Model file for the job. Use its own axes, mm. A direction names the side the tool comes from. Give positions to 0.01 mm unless a question says otherwise; leave off trailing zeros. Write each loop counter-clockwise with the first axis right and the second up, starting at its lowest first coordinate (ties: lowest second). Pieces come first, ordered by that corner, then holes.
```python
from build123d import *

# Parameters (mm, degrees)
BOSS_EXTRUDE1_DEPTH = 6.35
CUT_EXTRUDE1_DEPTH  = 64.001230115
FILLET2_R           = 3.81


with BuildPart() as part:
    # Sketch1 → Boss-Extrude1 (new body)
    with BuildSketch(Plane.XY):
        with BuildLine():
            Line((0, 47.625), (0, 36.83))
            ThreePointArc((0, 36.83), (36.83, 0), (0, -36.83))
            add(Edge.make_bspline(
                [(0, 47.625), (-26.600153249, 47.625), (-56.149642057, -0.404637175), (-24.15519568, -36.984078787), (0, -36.83)],
                knots=[0, 0, 0, 0, 0.529165327, 1, 1, 1, 1], degree=3))
        make_face()
        with BuildLine():
            Line((1.1176, -8.255), (8.255, -8.255))
            Line((8.255, -8.255), (8.255, -1.1176))
            Line((8.255, -1.1176), (9.657085657, -1.1176))
            ThreePointArc((9.657085657, -1.1176), (14.478, 0), (9.657085657, 1.1176))
            Line((9.657085657, 1.1176), (8.255, 1.1176))
            Line((8.255, 1.1176), (8.255, 8.255))
            Line((8.255, 8.255), (1.1176, 8.255))
            Line((1.1176, 8.255), (1.1176, 9.657085657))
            ThreePointArc((1.1176, 9.657085657), (0, 14.478), (-1.1176, 9.657085657))
            Line((-1.1176, 9.657085657), (-1.1176, 8.255))
            Line((-1.1176, 8.255), (-8.255, 8.255))
            Line((-8.255, 8.255), (-8.255, 1.1176))
            Line((-8.255, 1.1176), (-9.657085657, 1.1176))
            ThreePointArc((-9.657085657, 1.1176), (-14.478, 0), (-9.657085657, -1.1176))
            Line((-9.657085657, -1.1176), (-8.255, -1.1176))
            Line((-8.255, -1.1176), (-8.255, -8.255))
            Line((-8.255, -8.255), (-1.1176, -8.255))
            Line((-1.1176, -8.255), (-1.1176, -9.657085657))
            ThreePointArc((-1.1176, -9.657085657), (0, -14.478), (1.1176, -9.657085657))
            Line((1.1176, -9.657085657), (1.1176, -8.255))
        make_face(mode=Mode.SUBTRACT)
    extrude(amount=BOSS_EXTRUDE1_DEPTH)

    # Sketch5 → Cut-Extrude1 (cut, through all)
    with BuildSketch(Plane.XY.offset(6.35)):
        with BuildLine():
            ThreePointArc((-12.136378722, 32.883902073), (-23.899090909, 25.641297895), (-31.950108913, 14.416422734))
            ThreePointArc((-31.950108913, 14.416422734), (-28.392549398, 5.00872066), (-18.984847325, 8.566280175))
            ThreePointArc((-18.984847325, 8.566280175), (-14.200909091, 15.236133532), (-7.211471414, 19.539709927))
            ThreePointArc((-7.211471414, 19.539709927), (-3.001828995, 28.674259654), (-12.136378722, 32.883902073))
        make_face()
    extrude(amount=-CUT_EXTRUDE1_DEPTH, mode=Mode.SUBTRACT)

    # Fillet2
    fillet2_edges = [part.edges().sort_by_distance(p)[0] for p in [
        (0, 36.83, 3.175),
    ]]
    fillet(fillet2_edges, radius=FILLET2_R)


solid = part.part
```
1. Slice it at B-B, the plane z = 4.75. State how many separate pieces and enclosed holes the cut face has, and give its area (3 significant figures).
Calculated:
separate pieces: 1
enclosed holes: 2
area: 4,020 mm2
2. Pin check, flat tips, straight feed: P1, Ø2, axis at y = 10.5, z = 1.5, coming from the +X side; P2, Ø1.9, axis at y = 4, z = 4.5, coming from the -X side; P3, Ø0.7, axis at y = 9, z = 3.5, coming from the +X side. Stop position of each tip, or through.
Calculated:
P1: stops at x = 35.58
P2: stops at x = -40.75
P3: stops at x = 35.8
3. Probe probe 1 along X at (y, z) = (6.5, 2.5) (3 decimals); probe 2 along Y at (x, z) = (-4, 4.5) (3 decimals); probe 3 along Y at (x, z) = (-16.5, 3.5). List the from-to ranges inside material, lowest first.
Calculated:
probe 1: x = -40.626 to -30.534, -20.401 to -8.255, 8.255 to 36.252
probe 2: y = -36.693 to -8.255, 8.255 to 21.924, 30.5 to 47.429
probe 3: y = -33.86 to 12.71, 30.93 to 43.96
4. Pull direction Y, two halves, no side cores. Call faces 3 (the cylindrical face through (-0.095, -14.476, 3.131)), 4 (the flat face through (0, 44, 3)), 5 (the cylindrical face through (0.966, 37.926, 3.219)): +Y half, -Y half, draft (parallel to the pull), parting line (faces both ways), or undercut.
Calculated:
face 3: undercut
face 4: draft
face 5: +Y half
5. Slice it at A-A, the plane x = 13.5. Write the cut outline in (y, z), and give its area (3 significant figures).
Calculated:
outline: (-34.27, 0) - (-2, 0) - (-2, 6.35) - (-34.27, 6.35) - close; (2, 0) - (34.27, 0) - (34.27, 6.35) - (2, 6.35) - close
area: 410 mm2
6. Slice it at D-D, the plane x = 23. Write the cut outline in (y, z), and give its area (3 significant figures).
Calculated:
outline: (-28.77, 0) - (28.77, 0) - (28.77, 6.35) - (-28.77, 6.35) - close
area: 365 mm2
7. Which spindle directions (+Z, -Z, +X, -X, +Y, -Y) get a long thin tool onto all of the face, cutting with end or side? Do faces 1 (the flat face through (-9, -3, 6.35)), 2 (the flat face through (-5, 8.255, 3)). Say none if no direction does.
Calculated:
face 1: +Z, +X, -X, +Y, -Y
face 2: +Z, -Z
